from build123d import *

# Parameters (mm, degrees)
F1_DEPTH = 19.05


with BuildPart() as f1:
    # F0 (on Right) → F1 (new body)
    with BuildSketch(Plane.YZ):
        Polygon((19.05, 19.05), (19.05, 0), (228.6, 0), (228.6, 146.05), (0, 146.05), (0, 19.05), align=None)
        Polygon((19.05, 0), (0, 0), (-190.5, 0), (-190.5, -127), (228.6, -127), (228.6, 0), align=None)
    extrude(amount=F1_DEPTH)


solid = f1.part
Geometry: final body of the model. Coordinates: model frame, mm. A direction names the side the tool comes from. Give positions to 0.01 mm unless a question says otherwise; leave off trailing zeros. Write each loop counter-clockwise with the first axis right and the second up, starting at its lowest first coordinate (ties: lowest second). Pieces come first, ordered by that corner, then holes.
(1) Access query for faces 4 (the flat face through (9, 9, 19.05)), 5 (the flat face through (0, 63, -19)). Directions: +Z, -Z, +X, -X, +Y, -Y. A direction counts if a zero-diameter tool reaches every point of the face in a straight line with its end or side. Return the directions, or none.
(2) Cut plane B-B, the plane y = -59. Return loops of the section in (x, z).
(3) First-contact query: P1, Ø10, axis at y = -27, z = -47, coming from the -X side. Flat tip, straight axial feed; report the tip coordinate or a pass-through.
(4) Mould query, pull axis Z, two halves, no side actions, for faces 1 (the flat face through (9, 19.05, 10)), 2 (the flat face through (9, 16, -127)), 3 (the flat face through (9, 0, 83)). Classes: released by +Z, released by -Z, zero draft, split by the parting line, or undercut.
(5) Cut plane A-A, the plane x = 9.75. Return loops of the section in (y, z), then the cut area to 4 significant figures.
(6) Cut plane C-C, the plane z = 50.5. Return loops of the section in (x, y), then the cut area to 3 significant figures.
(7) Ray query, line 1 (Y direction, x = 18, z = 129.5); line 2 (Z direction, x = 16.5, y = 1); line 3 (Y direction, x = 14.25, z = 3). Return the intervals inside material, ascending.
Values follow:
1. face 4: +X, -X, -Y
1. face 5: +Z, -Z, -X, +Y, -Y
2. outline: (0, -127) - (19.05, -127) - (19.05, 0) - (0, 0) - close
3. P1: stops at x = 0
4. face 1: undercut
4. face 2: released by -Z
4. face 3: zero draft
5. outline: (-190.5, -127) - (228.6, -127) - (228.6, 146.05) - (0, 146.05) - (0, 19.05) - (19.05, 19.05) - (19.05, 0) - (-190.5, 0) - close
5. area: 86,250 mm2
6. outline: (0, 0) - (19.05, 0) - (19.05, 228.6) - (0, 228.6) - close
6. area: 4,350 mm2
7. line 1: y = 0 to 228.6
7. line 2: z = -127 to 0, 19.05 to 146.05
7. line 3: y = 19.05 to 228.6
